Source: three-view drawing plus pictorial views. Frame: mm from the lowest corner of the part. Give positions to 0.01 mm unless a question says otherwise; leave off trailing zeros. Loops run counter-clockwise (first coordinate to the right, second up) from the corner with the lowest first, then second, coordinate; pieces in that order, holes last. Notation, with made-up numbers: M 82,72.5 L 127,72.5 A25 cw 127,109.5 Z; hole C 66,18.5 d4. An arc over 180 degrees is marked long. One line per item, written item: value. Start each with the question number.
(1) Section B-B on y = 56.5. Output: boundary loops of the cut face in (x, z), plus the area to 3 significant figures.
(2) Pin query (flat end, axial travel): P1, Ø10.5, axis at x = 12.7, y = 63.5, coming from the -Z side; P2, Ø6, axis at x = 29.5, z = 4.5, coming from the +Y side. Return the tip coordinate at first contact, or that it passes through.
(3) Pull-direction query (X, two-part tool) for the marked faces 1, 2 and 3; classes: released by +X, released by -X, zero draft, split by the parting line, or undercut.
(4) Ray query, line 1 along Y through (x, z) = (139.7, 7) (1 decimal); line 2 along X through (y, z) = (11.5, 1.5); line 3 along X through (y, z) = (66, 7.5) (1 decimal). Return the intervals inside material, ascending. Write a range as from..to.
(5) Section A-A on x = 139.7. Output: boundary loops of the cut face in (y, z) (1 decimal).
(6) Section C-C on z = 3.5. Output: boundary loops of the cut face in (x, y) (1 decimal).
(7) Section D-D on y = 12.7. Output: boundary loops of the cut face in (x, z) (1 decimal), plus the area to 3 significant figures.
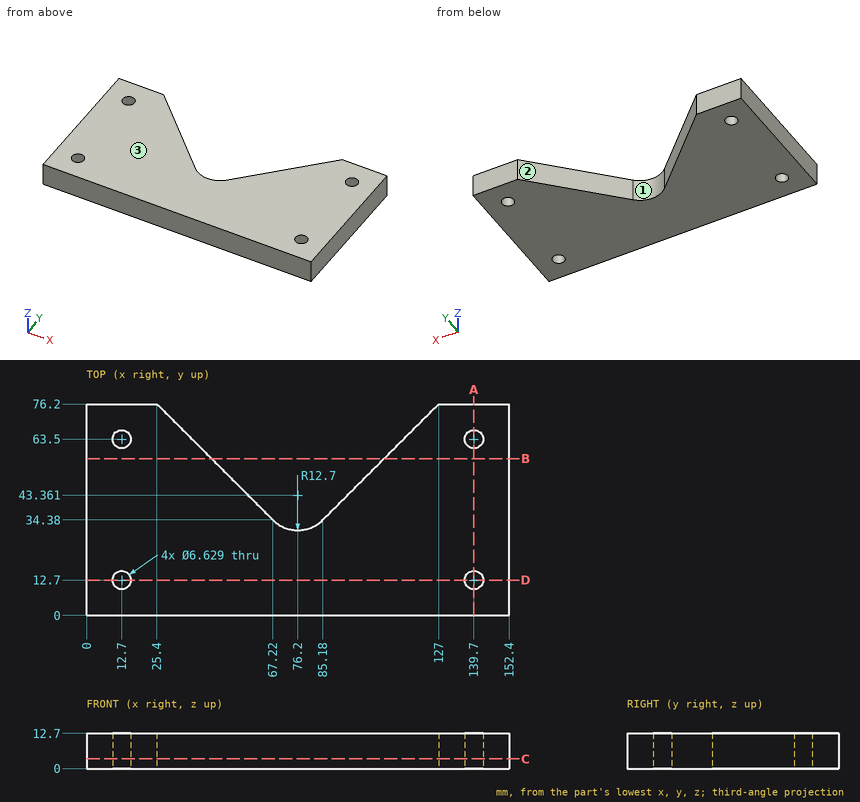
Output values:
1. outline: M 0,0 L 45.1,0 L 45.1,12.7 L 0,12.7 Z; M 107.3,0 L 152.4,0 L 152.4,12.7 L 107.3,12.7 Z
1. area: 1,150 mm²
2. P1: stops at z = 0
2. P2: stops at y = 75.1
3. face 1: undercut
3. face 2: undercut
3. face 3: zero draft
4. line 1: y = 0..9.4, 16..60.2, 66.8..76.2
4. line 2: x = 0..9.61, 15.79..136.61, 142.79..152.4
4. line 3: x = 0..10.5, 14.9..35.6, 116.8..137.5, 141.9..152.4
5. outline: M 0,0 L 9.4,0 L 9.4,12.7 L 0,12.7 Z; M 16,0 L 60.2,0 L 60.2,12.7 L 16,12.7 Z; M 66.8,0 L 76.2,0 L 76.2,12.7 L 66.8,12.7 Z
6. outline: M 0,0 L 152.4,0 L 152.4,76.2 L 127,76.2 L 85.2,34.4 A12.7 cw 67.2,34.4 L 25.4,76.2 L 0,76.2 Z; hole C 12.7,12.7 d6.6; hole C 12.7,63.5 d6.6; hole C 139.7,12.7 d6.6; hole C 139.7,63.5 d6.6
7. outline: M 0,0 L 9.4,0 L 9.4,12.7 L 0,12.7 Z; M 16,0 L 136.4,0 L 136.4,12.7 L 16,12.7 Z; M 143,0 L 152.4,0 L 152.4,12.7 L 143,12.7 Z
7. area: 1,770 mm²
